```python
from build123d import *

# Parameters (mm, degrees)
SKETCH1_R           = 10
SKETCH1_R_2         = 4.75
BOSS_EXTRUDE1_DEPTH = 10
CUT_EXTRUDE1_DEPTH  = 10


with BuildPart() as part:
    # Sketch1 → Boss-Extrude1 (new body)
    with BuildSketch(Plane(origin=(0, 0, 0), x_dir=(1, 0, 0), z_dir=(0, 1, 0))):
        Circle(SKETCH1_R)
        Circle(SKETCH1_R_2, mode=Mode.SUBTRACT)
    extrude(amount=BOSS_EXTRUDE1_DEPTH)

    # Sketch2 → Cut-Extrude1 (cut)
    with BuildSketch(Plane(origin=(10, 0, 0), x_dir=(0, 0, -1), z_dir=(1, 0, 0))):
        with BuildLine():
            ThreePointArc((0, 6.5), (-1.5, 5), (0, 3.5))
            Line((0, 3.5), (0, 6.5))
        make_face()
        with BuildLine():
            Line((0, 6.5), (0, 3.5))
            ThreePointArc((0, 3.5), (1.060660172, 3.939339828), (1.5, 5))
            ThreePointArc((1.5, 5), (1.060660172, 6.060660172), (0, 6.5))
        make_face()
    extrude(amount=-CUT_EXTRUDE1_DEPTH, mode=Mode.SUBTRACT)


solid = part.part
```
Geometry check sheet. Reference: the model listing, model coordinates, mm. Round coordinates to 2 decimals unless told otherwise and drop trailing zeros. Order: outer loops, then holes, each group sorted by start corner. A loop starts at its lowest first (then second) coordinate and runs counter-clockwise, first axis right, second up. Notation, with made-up numbers: (53.25, 37) -> (81.25, 37) arc R18 cw to (81.25, 47) -> close; hole circle Ø5 at (9.25, 16). An arc over 180 degrees is marked (long way). Return JSON: item names as keys, results as strings. Group by question number.
Q1. Section check D-D, the plane y = 1. Record the boundary of the cut face in (x, z), plus the area to 3 significant figures.
Q2. Section check C-C, the plane z = 0.5. Record the boundary of the cut face in (x, y), plus the area to 3 significant figures.
Q3. Release check for a two-part mould opening along Z. For faces 1 (the cylindrical face through (-3.77, 4.93, 2.89)), 2 (the cylindrical face through (-2.17, 4.93, 9.76)), 3 (the flat face through (-2.4, 10, 4.3)) record: released by +Z, released by -Z, zero draft, split by the parting line, or undercut.
Q4. Section check A-A, the plane x = 0. Record the boundary of the cut face in (y, z), plus the area to 3 significant figures.
Q5. Section check B-B, the plane x = 6. Record the boundary of the cut face in (y, z).
Q6. Material ranges on probe 1 along X at (y, z) = (2.5, 0); probe 2 along Y at (x, z) = (6.75, -0.25), recorded low to high. Write a range as from..to.
Q7. Gauge pin test, flat ends, axial feed: pin 1 (1 mm diameter, centred on y = 5.5, z = -5, fed in from +X); pin 2 (6 mm diameter, centred on x = 4.5, y = 5.5, fed in from -Z); pin 3 (4 mm diameter, centred on x = -0.5, y = 3.5, fed in from +Z); pin 4 (1.5 mm diameter, centred on x = 7, y = 1, fed in from -Z). Record the tip position at first contact, or that the pin passes through.
Numbers:
{
 "1": {"outline": "circle Ø20 at (0, 0); hole circle Ø9.5 at (0, 0)", "area": "243 mm^2"},
 "2": {"outline": "(-9.99, 0) -> (-4.72, 0) -> (-4.72, 10) -> (-9.99, 10) -> close; (4.72, 0) -> (9.99, 0) -> (9.99, 3.59) -> (4.72, 3.59) -> close; (4.72, 6.41) -> (9.99, 6.41) -> (9.99, 10) -> (4.72, 10) -> close", "area": "90.4 mm^2"},
 "3": {"face 1": "undercut", "face 2": "split by the parting line", "face 3": "zero draft"},
 "4": {"outline": "(0, -10) -> (10, -10) -> (10, -4.75) -> (0, -4.75) -> close; (0, 4.75) -> (10, 4.75) -> (10, 10) -> (0, 10) -> close", "area": "105 mm^2"},
 "5": {"outline": "(0, -8) -> (10, -8) -> (10, 8) -> (0, 8) -> close; hole circle Ø3 at (5, 0)"},
 "6": {"probe 1": "-10..-4.75, 4.75..10", "probe 2": "0..3.52, 6.48..10"},
 "7": {"pin 1": "x = 8.93", "pin 2": "z = -9.89", "pin 3": "z = 10", "pin 4": "z = -7.81"}
}
